Source: CAD feature listing. Evaluate the final solid. Frame: model axes, mm. Face numbers are marked on the shaded views. A direction names the side the tool comes from. Round coordinates to 2 decimals unless told otherwise and drop trailing zeros. Loops run counter-clockwise (first coordinate to the right, second up) from the corner with the lowest first, then second, coordinate; pieces in that order, holes last. Notation, with made-up numbers: M 54.25,73.25 L 66.25,73.25 A29 ccw 66.25,93.25 Z; hole C 42,53 d1. An arc over 180 degrees is marked long. Write each question's results on one line, items separated by ' | '. Start each with the question number.
1. Draft query along X for the marked faces 3, 4, 5 and 6. Return one class per face: released by +X, released by -X, zero draft, split by the parting line, or undercut.
2. Section A-A on x = 15.5. Output: boundary loops of the cut face in (y, z), and give its area (3 significant figures).
3. Ray query, line 1 (Y direction, x = 6.5, z = 2.5); line 2 (X direction, y = 8.25, z = 1.3); line 3 (X direction, y = 1.25, z = 1.2). Return the intervals inside material, ascending.
4. Section C-C on y = 4. Output: boundary loops of the cut face in (x, z), and give its area (3 significant figures).
5. Set-up query: the marked faces 1 and 2. Return all of +Z, -Z, +X, -X, +Y, -Y with unobstructed straight access to the full face (end or side cutting, diameter ignored); none if empty.
6. Section B-B on z = 3.05. Output: boundary loops of the cut face in (x, y), and give its area (3 significant figures).
from build123d import *

# Parameters (mm, degrees)
ESQUISSE1_W        = 20
ESQUISSE1_H        = 14.5
BOSS_EXTRU_1_DEPTH = 5


with BuildPart() as part:
    # Esquisse1 → Boss.-Extru.1 (new body)
    with BuildSketch(Plane.XY):
        with Locations((10, 7.25)):
            Rectangle(ESQUISSE1_W, ESQUISSE1_H)
        Polygon((17.274613392, 7.25), (13.637306696, 13.55), (6.362693304, 13.55), (2.725386608, 7.25), (6.362693304, 0.95), (13.637306696, 0.95), align=None, mode=Mode.SUBTRACT)
    extrude(amount=BOSS_EXTRU_1_DEPTH)


solid = part.part
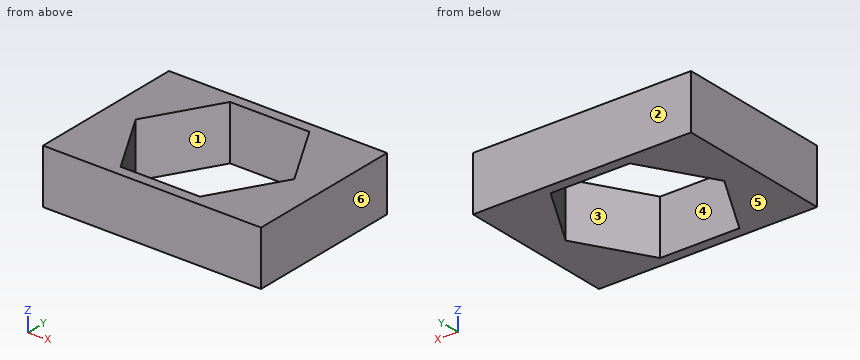
Taken from the geometry:
1) face 3: undercut | face 4: undercut | face 5: zero draft | face 6: released by +X
2) outline: M 0,0 L 4.18,0 L 4.18,5 L 0,5 Z; M 10.32,0 L 14.5,0 L 14.5,5 L 10.32,5 Z | area: 41.8 mm^2
3) line 1: 0 to 0.95, 13.55 to 14.5 | line 2: 0 to 3.3, 16.7 to 20 | line 3: 0 to 6.19, 13.81 to 20
4) outline: M 0,0 L 4.6,0 L 4.6,5 L 0,5 Z; M 15.4,0 L 20,0 L 20,5 L 15.4,5 Z | area: 46.0 mm^2
5) face 1: +Z, -Z | face 2: +Z, -Z, +X, -X, +Y
6) outline: M 0,0 L 20,0 L 20,14.5 L 0,14.5 Z; hole M 2.73,7.25 L 6.36,0.95 L 13.64,0.95 L 17.27,7.25 L 13.64,13.55 L 6.36,13.55 Z | area: 153 mm^2
